Source: CAD feature listing. Evaluate the final solid. Frame: model axes, mm. Face numbers are marked on the shaded views. A direction names the side the tool comes from. Round coordinates to 2 decimals unless told otherwise and drop trailing zeros. Write each loop counter-clockwise with the first axis right and the second up, starting at its lowest first coordinate (ties: lowest second). Pieces come first, ordered by that corner, then holes.
from build123d import *

# Parameters (mm, degrees)
SKETCH1_R           = 15
BOSS_EXTRUDE1_DEPTH = 3
SKETCH3_W           = 3.1
SKETCH3_H           = 11
CUT_EXTRUDE1_DEPTH  = 3


with BuildPart() as part:
    # Sketch1 → Boss-Extrude1 (new body)
    with BuildSketch(Plane.XY):
        Circle(SKETCH1_R)
    extrude(amount=BOSS_EXTRUDE1_DEPTH)

    # Sketch3 → Cut-Extrude1 (cut)
    with BuildSketch(Plane.XY):
        Rectangle(SKETCH3_W, SKETCH3_H)
    extrude(amount=CUT_EXTRUDE1_DEPTH, mode=Mode.SUBTRACT)


solid = part.part
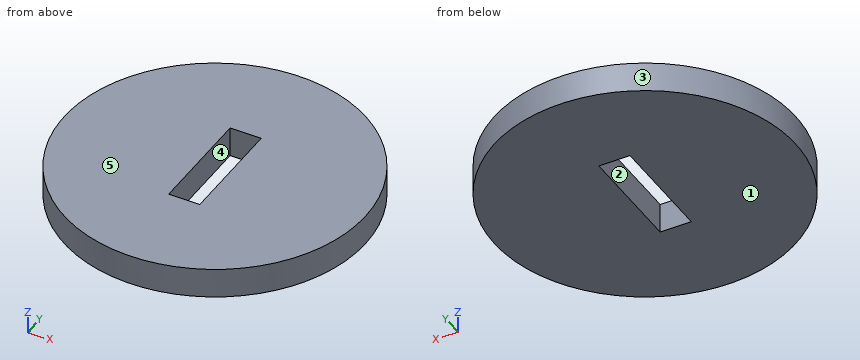
1) Reachability of the marked faces 1 and 2 from +Z, -Z, +X, -X, +Y, -Y: full face, straight path, thin tool, end or side. Return the list, or none.
Taken from the geometry:
face 1: -Z, +X, -X, +Y, -Y
face 2: +Z, -Z
2) Pull-direction query (X, two-part tool) for the marked faces 3, 4 and 5; classes: released by +X, released by -X, zero draft, split by the parting line, or undercut.
Taken from the geometry:
face 3: split by the parting line
face 4: undercut
face 5: zero draft
3) Section query C-C on z = 1.2. Return the cut outline in (x, y).
Taken from the geometry:
outline: circle Ø30 at (0, 0); hole (-1.55, -5.5) - (1.55, -5.5) - (1.55, 5.5) - (-1.55, 5.5) - close
4) Section query A-A on y = 0. Return the cut outline in (x, z).
Taken from the geometry:
outline: (-15, 0) - (-1.55, 0) - (-1.55, 3) - (-15, 3) - close; (1.55, 0) - (15, 0) - (15, 3) - (1.55, 3) - close
5) Section query D-D on x = 12. Return the cut outline in (y, z), then the cut area to 3 significant figures.
Taken from the geometry:
outline: (-9, 0) - (9, 0) - (9, 3) - (-9, 3) - close
area: 54.0 mm2
6) Contact query for flat-ended pins moving along their axis: P1, Ø1.5, axis at y = 2.5, z = 1.5, coming from the -X side; P2, Ø0.9, axis at y = -2, z = 2, coming from the +X side. Output: stop coordinate, or through.
Taken from the geometry:
P1: stops at x = -14.9
P2: stops at x = 14.92
7) Section query B-B on x = 0. Return the cut outline in (y, z), then the cut area to 3 significant figures.
Taken from the geometry:
outline: (-15, 0) - (-5.5, 0) - (-5.5, 3) - (-15, 3) - close; (5.5, 0) - (15, 0) - (15, 3) - (5.5, 3) - close
area: 57.0 mm2
8) Material intervals for line 1 (X direction, y = 2.25, z = 0.2); line 2 (X direction, y = 1, z = 0.9); line 3 (Y direction, x = -10.75, z = 0.4), sorted ascending.
Taken from the geometry:
line 1: x = -14.83 to -1.55, 1.55 to 14.83
line 2: x = -14.97 to -1.55, 1.55 to 14.97
line 3: y = -10.46 to 10.46
